Autodesk Inventor part; units mm, degrees
ref_plane "Work Plane1" through (0, 0.02, 0) normal (0, -1, 0) x (1, 0, 0)
ref_plane "Work Plane2" through (0, 1.105, 0) normal (0, 1, 0) x (1, 0, 0)
ref_plane "YZ Plane" through (0, 0, 0) normal (1, 0, 0) x (0, 1, 0)
sketch "Sketch2" plane through (0, 0, 0) normal (0, 1, 0) x (-1, 0, 0)
  line L0 (-25.3, 47.42) -> (25.3, 47.42)
  line L1 (29.3, 43.42) -> (29.3, -40.92)
  line L2 (22.8, -47.42) -> (-22.8, -47.42)
  line L3 (-29.3, -40.92) -> (-29.3, 43.42)
  arc A0 (-25.3, 47.42) -> (-29.3, 43.42) centre (-25.3, 43.42) ccw
  arc A1 (29.3, 43.42) -> (25.3, 47.42) centre (25.3, 43.42) ccw
  arc A2 (22.8, -47.42) -> (29.3, -40.92) centre (22.8, -40.92) ccw
  arc A3 (-29.3, -40.92) -> (-22.8, -47.42) centre (-22.8, -40.92) ccw
  point P0 (0, 0)
  point P1 (-29.3, 47.42)
  point P2 (29.3, -47.42)
  point P3 (29.3, 47.42)
  dimension "d6" = 94.84
  dimension "d7" = 58.6
  dimension "d8" = 29.3
  dimension "d9" = 47.42
  dimension "d23" = 4
  dimension "d24" = 4
  dimension "d25" = 6.5
  dimension "d26" = 6.5
extrude "Extrusion2" add sketch "Sketch2" along normal blind 1.125
sketch "Sketch1" plane through (0, 0, 0) normal (0, 1, 0) x (-1, 0, 0)
  line L0 (24.78, 37.02) -> (-24.78, 37.02)
  line L1 (-24.78, 37.02) -> (-24.78, -37.02)
  line L2 (-24.78, -37.02) -> (24.78, -37.02)
  line L3 (24.78, -37.02) -> (24.78, 37.02)
  point P0 (0, 0)
  dimension "d0" = 49.56
  dimension "d1" = 74.04
  dimension "d2" = 37.02
  dimension "d3" = 24.78
extrude "Extrusion1" cut sketch "Sketch1" along normal blind 1.3
ref_plane "Work Plane1" through (0, 0.02, 0) normal (0, -1, 0) x (1, 0, 0)
ref_plane "Work Plane2" through (0, 1.105, 0) normal (0, 1, 0) x (1, 0, 0)
sketch "Sketch4" plane through (0, 1.105, 0) normal (0, 1, 0) x (1, 0, 0)
  line L0 (-24.78, -37.02) -> (-24.78, 37.02)
  line L1 (24.78, -37.02) -> (-24.78, -37.02)
  line L2 (24.78, 37.02) -> (24.78, -37.02)
  line L3 (-24.78, 37.02) -> (24.78, 37.02)
  line L4 (-24.78, -37.02) -> (-24.78, 37.02)
  line L5 (-24.78, 37.02) -> (24.78, 37.02)
  line L6 (24.78, 37.02) -> (24.78, -37.02)
  line L7 (24.78, -37.02) -> (-24.78, -37.02)
  line L8 (29.3, -43.42) -> (29.3, 40.92)
  arc A0 (29.3, 40.92) -> (22.8, 47.42) centre (22.8, 40.92) ccw
  line L9 (22.8, 47.42) -> (-22.8, 47.42)
  arc A1 (-22.8, 47.42) -> (-29.3, 40.92) centre (-22.8, 40.92) ccw
  line L10 (-29.3, 40.92) -> (-29.3, -43.42)
  arc A2 (-29.3, -43.42) -> (-25.3, -47.42) centre (-25.3, -43.42) ccw
  line L11 (-25.3, -47.42) -> (25.3, -47.42)
  arc A3 (25.3, -47.42) -> (29.3, -43.42) centre (25.3, -43.42) ccw
  line L12 (-24.78, -37.02) -> (24.78, -37.02)
  line L13 (-24.78, -37.02) -> (24.78, -37.02)
  line L14 (24.78, -37.02) -> (24.78, 37.02)
  line L15 (24.78, 37.02) -> (-24.78, 37.02)
  line L16 (-24.78, 37.02) -> (-24.78, -37.02)
  point P0 (0, 0)
extrude "Extrusion4" add sketch "Sketch4" along normal up to surface (1.085 mm away) from surface at -1.085 contours L0 L3 L2 L1
equation "\"d24\" = d23"
equation "\"d26\" = d25"
properties part number "Touchcreen+Cover"
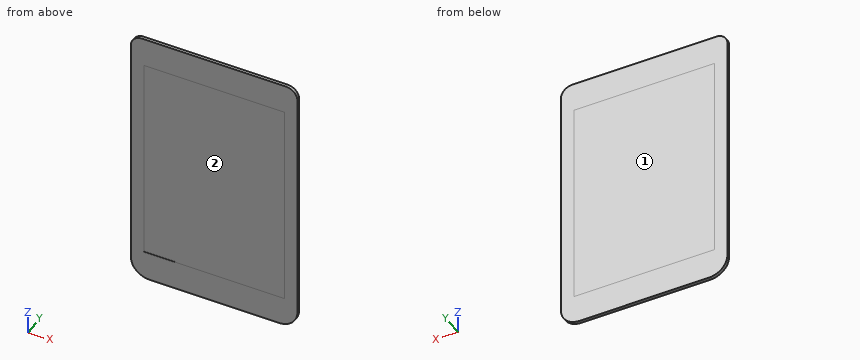
The listing builds one solid part. Answer for the finished solid, in the listing's coordinates (mm). Face numbers are marked on the shaded views. Coordinates: 2 decimals unless noted, no trailing zeros. Write each loop counter-clockwise with the first axis right and the second up, starting at its lowest first coordinate (ties: lowest second). Pieces come first, ordered by that corner, then holes. Notation, with made-up numbers: (75, 49) - (111, 49) arc R27 cw to (111, 68) - close; hole circle Ø7 at (78, 23). An arc over 180 degrees is marked (long way). Return JSON: item names as keys, results as strings.
1. The part is cut by section B-B on x = -21.5. Determine the outline of the cut face in (y, z) (3 decimals), then the cut area to 3 significant figures.
Final values:
{"outline": "(0, -47.42) - (1.125, -47.42) - (1.125, -37.02) - (1.105, -37.02) - (1.105, 37.02) - (1.125, 37.02) - (1.125, 47.42) - (0, 47.42) - (0, 37.02) - (0.02, 37.02) - (0.02, -37.02) - (0, -37.02) - close", "area": "104 mm^2"}
2. The part is cut by section A-A on z = 25. Determine the outline of the cut face in (x, y) (3 decimals), then the cut area to 3 significant figures.
Final values:
{"outline": "(-29.3, 0) - (-24.78, 0) - (-24.78, 0.02) - (24.78, 0.02) - (24.78, 0) - (29.3, 0) - (29.3, 1.125) - (24.78, 1.125) - (24.78, 1.105) - (-24.78, 1.105) - (-24.78, 1.125) - (-29.3, 1.125) - close", "area": "63.9 mm^2"}
3. Consider line 1 along Y through (x, z) = (-12.5, -1) (3 decimals); line 2 along Z through (x, y) = (24.5, 0.8); line 3 along Z through (x, y) = (-25.5, 0.55) (3 decimals). Determine where each line is inside the solid, lowest interval first.
Final values:
{"line 1": "0.02 to 1.105", "line 2": "-47.19 to 47.42", "line 3": "-46.833 to 47.415"}
4. This flat-tipped pin is pushed along its axis until it touches: pin 1 Ø5 at (x, z) = (2.5, -26) entering from -Y. Where does it stop, or does it pass through?
Final values:
{"pin 1": "y = 0.02"}
5. For a pull along Y with two mould halves and no side action, classify the marked faces 1 and 2 as +Y half, -Y half, draft (parallel to the pull), parting line (faces both ways), or undercut.
Final values:
{"face 1": "+Y half", "face 2": "-Y half"}
